The drawing under review shows one solid part. Ordinate dimensions are in mm from its lowest x, y, z. A direction names the side the tool comes from. Coordinates: 2 decimals unless noted, no trailing zeros. Write each loop counter-clockwise with the first axis right and the second up, starting at its lowest first coordinate (ties: lowest second). Pieces come first, ordered by that corner, then holes.
1) Add section A-A, the plane z = 7. State the section outline as (x, y) points.
2) Add section C-C, the plane x = 6. State the section outline as (y, z) points, then the cut area to 3 significant figures.
3) Machinability: for the marked faces 1, 2, 3 and 4, which of the approach directions +Z, -Z, +X, -X, +Y, -Y give a long, thin tool a straight path to every point of the face, cutting with its end or side? Answer none if there is none.
4) Add section D-D, the plane z = 26. State the section outline as (x, y) points, then the cut area to 3 significant figures.
5) For line 1 (X direction, y = 63, z = 6.5); line 2 (Z direction, x = 11, y = 76); line 3 (Z direction, x = 19.5, y = 32.5), list the stretches that pass through material, from the lowest coordinate up.
6) For P1, Ø16.5, axis at y = 5, z = 17, coming from the +X side; P2, Ø7.5, axis at x = 21.5, y = 6.5, coming from the +Z side; P3, Ø3, axis at x = 32.5, y = 60, coming from the -Z side, all flat-tipped, find the tip position at first contact; note any pin that passes through.
7) Mouldability with a two-part tool opening along X and no side actions: class the marked faces 5, 6 and 7 as released by +X, released by -X, zero draft, split by the parting line, or undercut.
8) Add section B-B, the plane y = 42. State the section outline as (x, z) points.
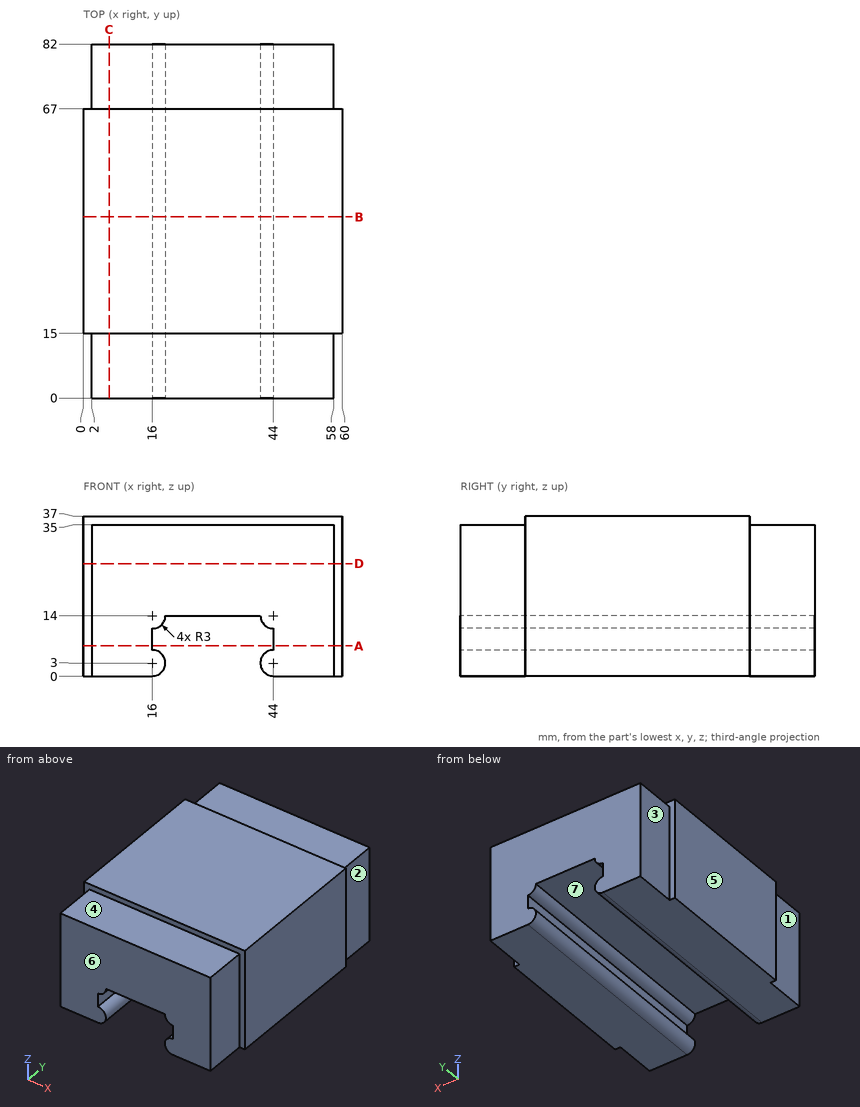
Geometry results:
1. outline: (0, 15) - (2, 15) - (2, 0) - (16, 0) - (16, 82) - (2, 82) - (2, 67) - (0, 67) - close; (44, 0) - (58, 0) - (58, 15) - (60, 15) - (60, 67) - (58, 67) - (58, 82) - (44, 82) - close
2. outline: (0, 0) - (82, 0) - (82, 35) - (67, 35) - (67, 37) - (15, 37) - (15, 35) - (0, 35) - close
2. area: 2,970 mm2
3. face 1: +Z, -Z, -X, -Y
3. face 2: +Z, -Z, +X, +Y
3. face 3: +Z, -Z, -X, +Y
3. face 4: +Z, +X, -X, -Y
4. outline: (0, 15) - (2, 15) - (2, 0) - (58, 0) - (58, 15) - (60, 15) - (60, 67) - (58, 67) - (58, 82) - (2, 82) - (2, 67) - (0, 67) - close
4. area: 4,800 mm2
5. line 1: x = 0 to 16, 44 to 60
5. line 2: z = 0 to 35
5. line 3: z = 14 to 37
6. P1: stops at x = 58
6. P2: stops at z = 35
6. P3: stops at z = 14
7. face 5: released by -X
7. face 6: zero draft
7. face 7: undercut
8. outline: (0, 0) - (16, 0) arc R3 ccw to (16, 6) - (16, 11) arc R3 ccw to (19, 14) - (41, 14) arc R3 ccw to (44, 11) - (44, 6) arc R3 ccw to (44, 0) - (60, 0) - (60, 37) - (0, 37) - close
